Source: CAD feature listing. Evaluate the final solid. Frame: model axes, mm. A direction names the side the tool comes from. Round coordinates to 2 decimals unless told otherwise and drop trailing zeros. Write each loop counter-clockwise with the first axis right and the second up, starting at its lowest first coordinate (ties: lowest second). Pieces come first, ordered by that corner, then holes. Notation, with made-up numbers: M -20.75,3.25 L 11.25,3.25 A17 cw 11.25,27.25 Z; hole C 3.5,18.25 d3. An arc over 180 degrees is marked long. Use a Markdown table: item, result.
```python
from build123d import *

# Parameters (mm, degrees)
SKETCH1_W            = 508
SKETCH1_H            = 304.8
BOSS_EXTRUDE1_DEPTH  = 25.4
SKETCH2_R            = 39.37
CUT_EXTRUDE1_DEPTH   = 12.7
LPATTERN1_COUNT      = 5
LPATTERN1_PITCH      = 101.6
LPATTERN1_COUNT_DIR2 = 3
LPATTERN1_PITCH_DIR2 = 101.6


with BuildPart() as part:
    # Sketch1 → Boss-Extrude1 (new body)
    with BuildSketch(Plane(origin=(0, 0, 0), x_dir=(1, 0, 0), z_dir=(0, 1, 0))):
        Rectangle(SKETCH1_W, SKETCH1_H)
    extrude(amount=BOSS_EXTRUDE1_DEPTH)

    # Sketch2 → Cut-Extrude1 (cut)
    with BuildSketch(Plane(origin=(0, 25.4, 0), x_dir=(1, 0, 0), z_dir=(0, 1, 0))):
        with Locations(Location((-203.2, -101.6, 0), (0, 0, 270))):
            Circle(SKETCH2_R)
    cut_extrude1 = extrude(amount=-CUT_EXTRUDE1_DEPTH, mode=Mode.SUBTRACT)

    # LPattern1: Cut-Extrude1 5 × 3
    with Locations(*[(i * LPATTERN1_PITCH, 0, -j * LPATTERN1_PITCH_DIR2) for i in range(LPATTERN1_COUNT) for j in range(LPATTERN1_COUNT_DIR2) if (i, j) != (0, 0)]):
        add(cut_extrude1, mode=Mode.SUBTRACT)


solid = part.part
```
Q1. Mould query, pull axis Z, two halves, no side actions, for faces 3 (the cylindrical face through (168.272, 19.139, 119.767)), 4 (the flat face through (-254, 13, 2)). Classes: +Z half, -Z half, draft (parallel to the pull), parting line (faces both ways), or undercut.
Results are:
| item | result |
|---|---|
| face 3 | undercut |
| face 4 | draft |
Q2. Section A-A on y = 19.25. Give the number of separate pieces and of enclosed holes in the cut face, plus the area to 3 significant figures.
Results are:
| item | result |
|---|---|
| separate pieces | 1 |
| enclosed holes | 15 |
| area | 81,800 mm^2 |
Q3. Section B-B on z = 101.6. Return loops of the section in (x, y), plus the area to 3 significant figures.
Results are:
| item | result |
|---|---|
| outline | M -254,0 L 254,0 L 254,25.4 L 242.57,25.4 L 242.57,12.7 L 163.83,12.7 L 163.83,25.4 L 140.97,25.4 L 140.97,12.7 L 62.23,12.7 L 62.23,25.4 L 39.37,25.4 L 39.37,12.7 L -39.37,12.7 L -39.37,25.4 L -62.23,25.4 L -62.23,12.7 L -140.97,12.7 L -140.97,25.4 L -163.83,25.4 L -163.83,12.7 L -242.57,12.7 L -242.57,25.4 L -254,25.4 Z |
| area | 7,900 mm^2 |
Q4. Reachability of faces 1 (the flat face through (-4, 0, -2)), 2 (the cylindrical face through (-34.928, 19.139, -83.433)) from +Z, -Z, +X, -X, +Y, -Y: full face, straight path, thin tool, end or side. Return the list, or none.
Results are:
| item | result |
|---|---|
| face 1 | +Z, -Z, +X, -X, -Y |
| face 2 | +Y |
Q5. Section C-C on x = -101.6. Return loops of the section in (y, z), plus the area to 3 significant figures.
Results are:
| item | result |
|---|---|
| outline | M 0,-152.4 L 25.4,-152.4 L 25.4,-140.97 L 12.7,-140.97 L 12.7,-62.23 L 25.4,-62.23 L 25.4,-39.37 L 12.7,-39.37 L 12.7,39.37 L 25.4,39.37 L 25.4,62.23 L 12.7,62.23 L 12.7,140.97 L 25.4,140.97 L 25.4,152.4 L 0,152.4 Z |
| area | 4,740 mm^2 |
Q6. Line query: L1, parallel to X at y = 22.75, z = -101.6; L2, parallel to Z at x = -177.5, y = 24; L3, parallel to Z at x = -109.5, y = 17.75. Output: solid intervals per line, ascending.
Results are:
| item | result |
|---|---|
| L1 | -254 to -242.57, -163.83 to -140.97, -62.23 to -39.37, 39.37 to 62.23, 140.97 to 163.83, 242.57 to 254 |
| L2 | -152.4 to -131.42, -71.78 to -29.82, 29.82 to 71.78, 131.42 to 152.4 |
| L3 | -152.4 to -140.17, -63.03 to -38.57, 38.57 to 63.03, 140.17 to 152.4 |
Q7. First-contact query: pin 1 Ø10 at (x, z) = (133.5, -66) entering from -Y; pin 2 Ø23.5 at (x, z) = (-215, 95.5) entering from +Y. Flat tips, straight axial feed; report the tip coordinate or a pass-through.
Results are:
| item | result |
|---|---|
| pin 1 | y = 0 |
| pin 2 | y = 12.7 |
Q8. Section D-D on x = -208. Return loops of the section in (y, z).
Results are:
| item | result |
|---|---|
| outline | M 0,-152.4 L 25.4,-152.4 L 25.4,-140.68 L 12.7,-140.68 L 12.7,-62.52 L 25.4,-62.52 L 25.4,-39.08 L 12.7,-39.08 L 12.7,39.08 L 25.4,39.08 L 25.4,62.52 L 12.7,62.52 L 12.7,140.68 L 25.4,140.68 L 25.4,152.4 L 0,152.4 Z |
